from build123d import *

# Parameters (mm, degrees)
BOSS_EXTRUDE1_DEPTH = 19.05


with BuildPart() as part:
    # Sketch1 → Boss-Extrude1 (new body)
    with BuildSketch(Plane(origin=(0, 0, 0), x_dir=(1, 0, 0), z_dir=(0, 1, 0))):
        with BuildLine():
            Line((-37, -33.02), (-37, 0))
            Line((-37, 0), (37, 0))
            Line((37, 0), (37, -33.02))
            Line((37, -33.02), (56.05, -33.02))
            Line((56.05, -33.02), (56.05, -29.845))
            ThreePointArc((56.05, -29.845), (55.12006403, -27.59993597), (52.875, -26.67))
            Line((52.875, -26.67), (49.7, -26.67))
            ThreePointArc((49.7, -26.67), (45.209871939, -24.810128061), (43.35, -20.32))
            Line((43.35, -20.32), (43.35, 0))
            Line((43.35, 0), (43.35, 3.175))
            ThreePointArc((43.35, 3.175), (42.42006403, 5.42006403), (40.175, 6.35))
            Line((40.175, 6.35), (-40.175, 6.35))
            ThreePointArc((-40.175, 6.35), (-42.42006403, 5.42006403), (-43.35, 3.175))
            Line((-43.35, 3.175), (-43.35, 0))
            Line((-43.35, 0), (-43.35, -20.32))
            ThreePointArc((-43.35, -20.32), (-45.209871939, -24.810128061), (-49.7, -26.67))
            Line((-49.7, -26.67), (-52.875, -26.67))
            ThreePointArc((-52.875, -26.67), (-55.12006403, -27.59993597), (-56.05, -29.845))
            Line((-56.05, -29.845), (-56.05, -33.02))
            Line((-56.05, -33.02), (-37, -33.02))
        make_face()
    extrude(amount=BOSS_EXTRUDE1_DEPTH)


solid = part.part
The model under review builds one solid part; all positions refer to its coordinate system, in mm. A direction names the side the tool comes from. Round coordinates to 2 decimals unless told otherwise and drop trailing zeros. Loops run counter-clockwise (first coordinate to the right, second up) from the corner with the lowest first, then second, coordinate; pieces in that order, holes last. Notation, with made-up numbers: (74, 30) -> (124, 30) arc R33 ccw to (124, 58) -> close; hole circle Ø3 at (27, 77). An arc over 180 degrees is marked (long way). Write item = value, one per line. Start each with the question number.
Item 1: Take a section at C-C on x = 25.5. Give the boundary of the cut face in (y, z), plus the area to 3 significant figures.
Item 2: For faces 4 (the flat face through (43.35, 9, 9)), 5 (the flat face through (37, 9, 16)), 6 (the flat face through (0, 19.05, -1)), 7 (the flat face through (-43.35, 9, 8)), list the 3-axis set-ups (+Z, -Z, +X, -X, +Y, -Y) from which the entire face can be reached by the end or side of a thin tool; tool diameter is ignored.
Item 3: Take a section at A-A on z = 6. Give the boundary of the cut face in (x, y).
Item 4: Take a section at B-B on y = 8.25. Give the boundary of the cut face in (x, z) (3 decimals).
Item 5: Take a section at D-D on z = 24.5. Give the boundary of the cut face in (x, y), plus the area to 3 significant figures.
Item 6: Mouldability with a two-part tool opening along X and no side actions: class faces 1 (the flat face through (1, 9, -6.35)), 2 (the flat face through (-56.05, 9, 31)), 3 (the flat face through (-37, 9, 17)) as released by +X, released by -X, zero draft, split by the parting line, or undercut.
Item 7: To check wall thickness, follow L1, parallel to X at y = 1.75, z = 6.5; L2, parallel to X at y = 16.25, z = 23; L3, parallel to Z at x = 0.5, y = 11. State the ranges of each line that lie inside material, in increasing order.
Item 8: Insertion check: pin 1 (6 mm diameter, centred on x = 24, z = 2, fed in from -Y); pin 2 (5 mm diameter, centred on y = 5.5, z = 12, fed in from -X); pin 3 (5.5 mm diameter, centred on y = 14, z = 6.5, fed in from +X); pin 4 (1 mm diameter, centred on x = 51.5, y = 9, fed in from -Z). Each pin has a flat end and moves straight along its axis. Give the tip position at first contact, or say it passes through.
Result:
q1.outline = (0, -6.35) -> (19.05, -6.35) -> (19.05, 0) -> (0, 0) -> close
q1.area = 121 mm²
q2.face_4 = -Z, +X, +Y, -Y
q2.face_5 = +Z, +Y, -Y
q2.face_6 = +Z, -Z, +X, -X, +Y
q2.face_7 = -Z, -X, +Y, -Y
q3.outline = (-43.35, 0) -> (-37, 0) -> (-37, 19.05) -> (-43.35, 19.05) -> close; (37, 0) -> (43.35, 0) -> (43.35, 19.05) -> (37, 19.05) -> close
q4.outline = (-56.05, 29.845) arc R3.175 ccw to (-52.875, 26.67) -> (-49.7, 26.67) arc R6.35 cw to (-43.35, 20.32) -> (-43.35, -3.175) arc R3.175 ccw to (-40.175, -6.35) -> (40.175, -6.35) arc R3.175 ccw to (43.35, -3.175) -> (43.35, 20.32) arc R6.35 cw to (49.7, 26.67) -> (52.875, 26.67) arc R3.175 ccw to (56.05, 29.845) -> (56.05, 33.02) -> (37, 33.02) -> (37, 0) -> (-37, 0) -> (-37, 33.02) -> (-56.05, 33.02) -> close
q5.outline = (-44.92, 0) -> (-37, 0) -> (-37, 19.05) -> (-44.92, 19.05) -> close; (37, 0) -> (44.92, 0) -> (44.92, 19.05) -> (37, 19.05) -> close
q5.area = 302 mm²
q6.face_1 = zero draft
q6.face_2 = released by -X
q6.face_3 = undercut
q7.L1 = -43.35 to -37, 37 to 43.35
q7.L2 = -43.94 to -37, 37 to 43.94
q7.L3 = -6.35 to 0
q8.pin_1 = 0
q8.pin_2 = -43.35
q8.pin_3 = 43.35
q8.pin_4 = 26.67
